Here's how the part is built. I have some questions about the finished solid (model axes, mm). A direction names the side the tool comes from. Give positions to 0.01 mm unless a question says otherwise; leave off trailing zeros. Write each loop counter-clockwise with the first axis right and the second up, starting at its lowest first coordinate (ties: lowest second). Pieces come first, ordered by that corner, then holes. Notation, with made-up numbers: (39, 23) - (44, 23) arc R30 cw to (44, 62) - close; hole circle Ø7 at (-20, 64.5). An arc over 180 degrees is marked (long way). Use a Markdown table: item, result.
```python
from build123d import *

# Parameters (mm, degrees)
SKETCH1_R            = 20
BOSS_EXTRUDE1_DEPTH  = 15
SKETCH2_R            = 10
BOSS_EXTRUDE2_DEPTH  = 8
SKETCH3_R            = 15
BOSS_EXTRUDE3_DEPTH  = 30
CUT_EXTRUDE1_START   = -30
CUT_EXTRUDE1_DEPTH   = 30
CIRPATTERN1_COUNT    = 16
BOSS_EXTRUDE5_DEPTH  = 10
SKETCH9_R            = 20
BOSS_EXTRUDE6_DEPTH  = 30
BOSS_EXTRUDE7_DEPTH  = 10
BOSS_EXTRUDE8_DEPTH  = 10
BOSS_EXTRUDE9_REACH  = 168.067
SKETCH14_R           = 20
SKETCH15_R           = 20
BOSS_EXTRUDE10_DEPTH = 15
SKETCH16_R           = 10
BOSS_EXTRUDE11_DEPTH = 8


with BuildPart() as part:
    # Sketch1 → Boss-Extrude1 (new body)
    with BuildSketch(Plane.XY):
        Circle(SKETCH1_R)
    extrude(amount=BOSS_EXTRUDE1_DEPTH)

    # Sketch2 → Boss-Extrude2 (add)
    with BuildSketch(Plane.XY.offset(15)):
        Circle(SKETCH2_R)
    extrude(amount=BOSS_EXTRUDE2_DEPTH)

    # Sketch3 → Boss-Extrude3 (add)
    with BuildSketch(Plane.XY.offset(23)):
        Circle(SKETCH3_R)
    extrude(amount=BOSS_EXTRUDE3_DEPTH)

    # Sketch5 → Cut-Extrude1 (cut)
    with BuildSketch(Plane.XY.offset(53).offset(CUT_EXTRUDE1_START)):
        with BuildLine():
            ThreePointArc((3.157894737, 14.663822859), (1.587869189, 14.915718938), (0, 15))
            Line((0, 15), (0, 13.5))
            ThreePointArc((0, 13.5), (1.42908227, 13.424147044), (2.842105263, 13.197440573))
            Line((2.842105263, 13.197440573), (3.157894737, 14.663822859))
        make_face()
    cut_extrude1 = extrude(amount=CUT_EXTRUDE1_DEPTH, mode=Mode.SUBTRACT)

    # CirPattern1: Cut-Extrude1 ×16 about axis
    cirpattern1_axis = Axis((0, 0, 0), (0, 0, 1))
    for i in range(1, CIRPATTERN1_COUNT):
        add(cut_extrude1.rotate(cirpattern1_axis, i * 360 / CIRPATTERN1_COUNT), mode=Mode.SUBTRACT)

    # Sketch8 → Boss-Extrude5 (add)
    with BuildSketch(Plane(origin=(0, 0, 0), x_dir=(-1, 0, 0), z_dir=(0, 0, -1))):
        with BuildLine():
            ThreePointArc((70, 20), (0, 90), (-70, 20))
            ThreePointArc((-70, 20), (-72.432874235, -9.018340852), (-89.130077464, -32.875968295))
            ThreePointArc((-89.130077464, -32.875968295), (0, -95), (89.130077464, -32.875968295))
            ThreePointArc((89.130077464, -32.875968295), (72.432874235, -9.018340852), (70, 20))
        make_face()
    extrude(amount=BOSS_EXTRUDE5_DEPTH)

    # Sketch9 → Boss-Extrude6 (add)
    with BuildSketch(Plane(origin=(0, 0, -10), x_dir=(-1, 0, 0), z_dir=(0, 0, -1))):
        with Locations((0, 50)):
            Circle(SKETCH9_R)
    extrude(amount=BOSS_EXTRUDE6_DEPTH)

    # Sketch10 → Boss-Extrude7 (add)
    with BuildSketch(Plane(origin=(0, 0, -40), x_dir=(-1, 0, 0), z_dir=(0, 0, -1))):
        with BuildLine():
            ThreePointArc((-70, -20), (0, -90), (70, -20))
            ThreePointArc((70, -20), (72.432874235, 9.018340852), (89.130077464, 32.875968295))
            ThreePointArc((89.130077464, 32.875968295), (0, 95), (-89.130077464, 32.875968295))
            ThreePointArc((-89.130077464, 32.875968295), (-72.432874235, 9.018340852), (-70, -20))
        make_face()
    extrude(amount=BOSS_EXTRUDE7_DEPTH)


with BuildPart() as body_2:
    # Sketch12 → Boss-Extrude8 (new body)
    with BuildSketch(Plane(origin=(0, 0, -80), x_dir=(-1, 0, 0), z_dir=(0, 0, -1))):
        with BuildLine():
            ThreePointArc((70, 20), (0, 90), (-70, 20))
            ThreePointArc((-70, 20), (-72.432874235, -9.018340852), (-89.130077464, -32.875968295))
            ThreePointArc((-89.130077464, -32.875968295), (0, -95), (89.130077464, -32.875968295))
            ThreePointArc((89.130077464, -32.875968295), (72.432874235, -9.018340852), (70, 20))
        make_face()
    extrude(amount=BOSS_EXTRUDE8_DEPTH)

    # Sketch14 → Boss-Extrude9 (add, up to next)
    with BuildSketch(Plane(origin=(0, 0, -50), x_dir=(-1, 0, 0), z_dir=(0, 0, -1)), mode=Mode.PRIVATE) as boss_extrude9_sk1:
        with Locations((0, -50)):
            Circle(SKETCH14_R)
    boss_extrude9_tool1 = extrude(boss_extrude9_sk1.sketch, amount=BOSS_EXTRUDE9_REACH, mode=Mode.PRIVATE) - body_2.part

    add(part.part)  # Boss-Extrude9 merges part
    add(boss_extrude9_tool1.solids().sort_by_distance((0, -50, -50))[0])

    # Sketch15 → Boss-Extrude10 (add)
    with BuildSketch(Plane(origin=(0, 0, -90), x_dir=(-1, 0, 0), z_dir=(0, 0, -1))):
        with Locations(Location((0, 0, 0), (0, 0, 180))):
            Circle(SKETCH15_R)
    extrude(amount=BOSS_EXTRUDE10_DEPTH)

    # Sketch16 → Boss-Extrude11 (add)
    with BuildSketch(Plane(origin=(0, 0, -105), x_dir=(-1, 0, 0), z_dir=(0, 0, -1))):
        with Locations(Location((0, 0, 0), (0, 0, 180))):
            Circle(SKETCH16_R)
    extrude(amount=BOSS_EXTRUDE11_DEPTH)


solid = body_2.part
```
Item 1: If we section it at B-B, the plane x = -56.5: Write out the boundary of the cut face in (y, z), plus the area to 3 significant figures.
Values:
| item | result |
|---|---|
| outline | (-76.37, -90) - (61.32, -90) - (61.32, -80) - (-76.37, -80) - close; (-76.37, -10) - (61.32, -10) - (61.32, 0) - (-76.37, 0) - close; (-61.32, -50) - (76.37, -50) - (76.37, -40) - (-61.32, -40) - close |
| area | 4,130 mm2 |
Item 2: Thinking about a two-plate mould opening in Y: for faces 5 (the cylindrical face through (-1.539, 89.983, -4.93)), 6 (the cylindrical face through (72.575, 9.406, -44.93)), 7 (the cylindrical face through (72.294, -8.63, -84.93)), 8 (the flat face through (1, -22, 0)), which applies, +Y half, -Y half, draft (parallel to the pull), parting line (faces both ways), or undercut?
Values:
| item | result |
|---|---|
| face 5 | +Y half |
| face 6 | undercut |
| face 7 | undercut |
| face 8 | draft |
Item 3: If we section it at D-D, the plane z = -53: Write out the boundary of the cut face in (x, y).
Values:
| item | result |
|---|---|
| outline | circle Ø40 at (0, -50) |
Item 4: Will these pins go through, and if not, where does the flat tip stop? pin 1 Ø8 at (x, z) = (30, -93.5) entering from -Y; pin 2 Ø1.6 at (x, z) = (14.5, 43.5) entering from -Y; pin 3 Ø1.6 at (y, z) = (-14, 34) entering from -X.
Values:
| item | result |
|---|---|
| pin 1 | stops at y = -90.76 |
| pin 2 | stops at y = -5.74 |
| pin 3 | stops at x = -5.74 |
Item 5: I need wall thicknesses on line 1 along Z through (x, y) = (-56.5, 58); line 2 along Z through (x, y) = (-2.5, 3); line 3 along Z through (x, y) = (-45, -77). Which ranges of each line are inside material? Lowest first, please. Write a range as [from, to].
Values:
| item | result |
|---|---|
| line 1 | z = [-90, -80], [-50, -40], [-10, 0] |
| line 2 | z = [-113, -80], [-50, -40], [-10, 53] |
| line 3 | z = [-90, -80], [-10, 0] |
Item 6: For faces 1 (the cylindrical face through (-1.539, 89.983, -84.93)), 2 (the flat face through (-5, -9, -105)), 3 (the cylindrical face through (-72.575, -9.406, -84.93)), 4 (the cylindrical face through (-2.17, -9.76, 18.94)), which set-ups out of +Z, -Z, +X, -X, +Y, -Y let a thin tool reach every point of the face, with its end or its side?
Values:
| item | result |
|---|---|
| face 1 | -Z, +Y |
| face 2 | -Z |
| face 3 | -Z, -X |
| face 4 | none |
Item 7: If we section it at C-C, the plane y = -50: Write out the boundary of the cut face in (x, z), plus the area to 3 significant figures.
Values:
| item | result |
|---|---|
| outline | (-80.78, -90) - (80.78, -90) - (80.78, -80) - (20, -80) - (20, -50) - (63.25, -50) - (63.25, -40) - (-63.25, -40) - (-63.25, -50) - (-20, -50) - (-20, -80) - (-80.78, -80) - close; (-80.78, -10) - (80.78, -10) - (80.78, 0) - (-80.78, 0) - close |
| area | 5,700 mm2 |
Item 8: If we section it at A-A, the plane y = -82: Write out the boundary of the cut face in (x, z), plus the area to 3 significant figures.
Values:
| item | result |
|---|---|
| outline | (-47.97, -90) - (47.97, -90) - (47.97, -80) - (-47.97, -80) - close; (-47.97, -10) - (47.97, -10) - (47.97, 0) - (-47.97, 0) - close; (-32.5, -50) - (32.5, -50) - (32.5, -40) - (-32.5, -40) - close |
| area | 2,570 mm2 |
